Geometry check sheet. Reference: the model listing, model coordinates, mm. Face numbers are marked on the shaded views. Round coordinates to 2 decimals unless told otherwise and drop trailing zeros. Order: outer loops, then holes, each group sorted by start corner. A loop starts at its lowest first (then second) coordinate and runs counter-clockwise, first axis right, second up.
(1) Sectioned sample at A-A (x = 0). Record the boundary of the cut face in (y, z), plus the area to 3 significant figures.
(2) Material ranges on line 1 along Y through (x, z) = (0, 4.5); line 2 along Y through (x, z) = (-1.25, 2.75); line 3 along X through (y, z) = (2, 6.5), recorded low to high.
(3) Go/stop test with flat-tipped pins: pin 1 (1 mm diameter, centred on y = 2.5, z = 6, fed in from +X); pin 2 (2 mm diameter, centred on y = -2, z = 4, fed in from -X). Record where each tip stops, or that it passes through.
(4) Release check for a two-part mould opening along Z. For the marked faces 1, 2 and 3 record: +Z half, -Z half, draft (parallel to the pull), parting line (faces both ways), or undercut.
from build123d import *

# Parameters (mm, degrees)
SKETCH1_R                                       = 7.105443578
SKETCH1_R_2                                     = 3
BOSS_EXTRUDE3_DEPTH                             = 8
CSK_FOR_M2_FLAT_HEAD_MACHINE_SCREW2_D           = 2.4
CSK_FOR_M2_FLAT_HEAD_MACHINE_SCREW2_CSINK_D     = 4.4
CSK_FOR_M2_FLAT_HEAD_MACHINE_SCREW2_CSINK_ANGLE = 90


with BuildPart() as part:
    # Sketch1 → Boss-Extrude3 (new body)
    with BuildSketch(Plane.XY):
        Circle(SKETCH1_R)
        Circle(SKETCH1_R_2, mode=Mode.SUBTRACT)
    extrude(amount=BOSS_EXTRUDE3_DEPTH)

    # CSK for M2 Flat Head Machine Screw2 (through all)
    with Locations(Plane(origin=(5.371974404, -4.650722466, 3.893731666), x_dir=(0.654529504622, 0.75603645916, 0), z_dir=(0.75603645916, -0.654529504622, 0))):
        with Locations((0, 0)):
            CounterSinkHole(CSK_FOR_M2_FLAT_HEAD_MACHINE_SCREW2_D / 2, CSK_FOR_M2_FLAT_HEAD_MACHINE_SCREW2_CSINK_D / 2, counter_sink_angle=CSK_FOR_M2_FLAT_HEAD_MACHINE_SCREW2_CSINK_ANGLE)


solid = part.part
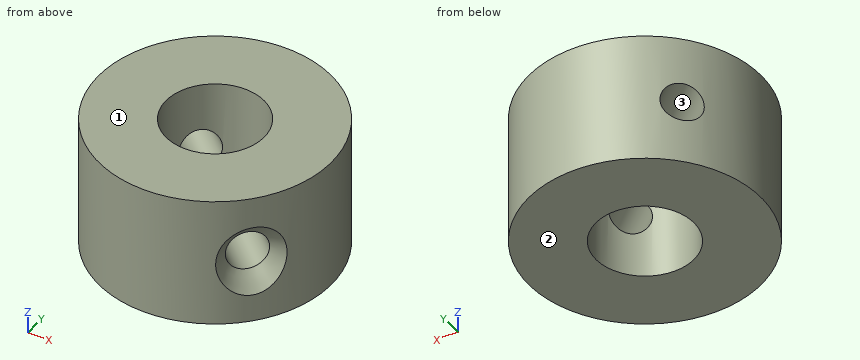
Answer below:
1. outline: (-7.11, 0) - (-3, 0) - (-3, 8) - (-7.11, 8) - close; (3, 0) - (7.11, 0) - (7.11, 8) - (3, 8) - close
1. area: 65.7 mm2
2. line 1: y = -7.11 to -3, 3 to 7.11
2. line 2: y = -6.99 to -2.73, 2.73 to 6.99
2. line 3: x = -6.82 to -2.24, 2.24 to 6.82
3. pin 1: stops at x = 6.82
3. pin 2: stops at x = -7.03
4. face 1: +Z half
4. face 2: -Z half
4. face 3: undercut
